Autodesk Inventor part; units mm, degrees
ref_plane "YZ Plane" through (0, 0, 0) normal (1, 0, 0) x (0, 1, 0)
ref_plane "XZ Plane" through (0, 0, 0) normal (0, 1, 0) x (-1, 0, 0)
ref_plane "XY Plane" through (0, 0, 0) normal (0, 0, 1) x (1, 0, 0)
sketch "Sketch1" plane through (0, 0, 0) normal (0, 0, 1) x (1, 0, 0)
  circle A0 centre (0, 0) radius 6.15
  line L0 (-4.2968, 4.4) -> (-16.8146, 2.7257)
  arc A1 (-16.8146, 2.7257) -> (-16.8146, -2.7257) centre (-16.45, 0) ccw
  line L1 (-16.8146, -2.7257) -> (-4.2968, -4.4)
  line L2 (4.2968, -4.4) -> (16.8146, -2.7257)
  arc A2 (16.8146, -2.7257) -> (16.8146, 2.7257) centre (16.45, 0) ccw
  line L3 (16.8146, 2.7257) -> (4.2968, 4.4)
  line L4 (-4.2968, -4.4) -> (4.2968, -4.4) construction
  line L5 (-4.2968, 4.4) -> (4.2968, 4.4) construction
  line L6 (-19.2, 0) -> (19.2, 0) construction
  circle A3 centre (0, 0) radius 11.25
  point P0 (-10.6763, 3.5467)
  point P1 (-10.6763, -3.5467)
  point P2 (10.6763, 3.5467)
  point P3 (10.6763, -3.5467)
  dimension "d0" = 12.3
  dimension "d1" = 8.8
  dimension "d2" = 38.4
  dimension "d3" = 2.75
  dimension "d10" = 22.5
extrude "Extrusion1" add sketch "Sketch1" along normal blind 2.3 contours A0 | A0 L3 A3 L2 | A0 L1 A3 L0
sketch "Sketch2" plane through (0, 0, 2.3) normal (0, 0, 1) x (1, 0, 0)
  circle A0 centre (0, 0) radius 4.4
  circle A1 centre (0, 0) radius 2.85
  dimension "d6" = 8.8
  dimension "d7" = 5.7
extrude "Extrusion2" add sketch "Sketch2" along normal blind 3.3
properties part number "attachment_real" material "Nylon 6/6"
Geometry: final body of the model. Coordinates: model frame, mm. A direction names the side the tool comes from. Coordinates: 2 decimals unless noted, no trailing zeros. Loops run counter-clockwise (first coordinate to the right, second up) from the corner with the lowest first, then second, coordinate; pieces in that order, holes last. Notation, with made-up numbers: (-38, 14) - (5, 14) arc R17 ccw to (5, 32) - close; hole circle Ø11 at (88, 88.25). An arc over 180 degrees is marked (long way). Put each result on its own line as item: value. Start each with the question number.
Q1. Cut plane A-A, the plane z = 5.05. Return loops of the section in (x, y).
Q2. Pull-direction query (Y, two-part tool) for faces 1 (the flat face through (1, -3, 5.6)), 2 (the flat face through (0, 0, 2.3)), 3 (the cylindrical face through (-0.07, 6.15, 1.13)), 4 (the cylindrical face through (-11.25, -0.05, 1.13)); classes: released by +Y, released by -Y, zero draft, split by the parting line, or undercut.
Q3. Pin query (flat end, axial travel): pin 1 Ø4 at (x, y) = (-8.5, -0.5) entering from -Z; pin 2 Ø1.5 at (x, z) = (4.5, 4) entering from +Y; pin 3 Ø2 at (x, z) = (5, 2.5) entering from -Y; pin 4 Ø2 at (x, z) = (6, 2) entering from +Y. Return the tip coordinate at first contact, or that it passes through.
Q4. Set-up query: faces 5 (the flat face through (7.44, -3.98, 1.13)), 6 (the cylindrical face through (4.197, -1.322, 3.927)). Return all of +Z, -Z, +X, -X, +Y, -Y with unobstructed straight access to the full face (end or side cutting, diameter ignored); none if empty.
Q5. Cut plane C-C, the plane y = 0. Return loops of the section in (x, z).
Q6. Cut plane D-D, the plane x = -3.5. Return loops of the section in (y, z), and give its area (3 significant figures).
Q7. Line query: line 1 (Y direction, x = 0, z = 4.7); line 2 (Z direction, x = -7.5, y = 3.25); line 3 (X direction, y = 1, z = 5.3). Output: solid intervals per line, ascending.
Q8. Cut plane B-B, the plane x = 0. Return loops of the section in (y, z).
Filled sheet:
1. outline: circle Ø8.8 at (0, 0); hole circle Ø5.7 at (0, 0)
2. face 1: zero draft
2. face 2: undercut
2. face 3: released by +Y
2. face 4: split by the parting line
3. pin 1: z = 0
3. pin 2: y = 2.3
3. pin 3: y = -4.65
3. pin 4: y = 4.31
4. face 5: +Z, -Z, +X, -Y
4. face 6: +Z
5. outline: (-11.25, 0) - (11.25, 0) - (11.25, 2.3) - (4.4, 2.3) - (4.4, 5.6) - (2.85, 5.6) - (2.85, 2.3) - (-2.85, 2.3) - (-2.85, 5.6) - (-4.4, 5.6) - (-4.4, 2.3) - (-11.25, 2.3) - close
6. outline: (-5.06, 0) - (5.06, 0) - (5.06, 2.3) - (2.67, 2.3) - (2.67, 5.6) - (-2.67, 5.6) - (-2.67, 2.3) - (-5.06, 2.3) - close
6. area: 40.9 mm²
7. line 1: -4.4 to -2.85, 2.85 to 4.4
7. line 2: 0 to 2.3
7. line 3: -4.28 to -2.67, 2.67 to 4.28
8. outline: (-6.15, 0) - (6.15, 0) - (6.15, 2.3) - (4.4, 2.3) - (4.4, 5.6) - (2.85, 5.6) - (2.85, 2.3) - (-2.85, 2.3) - (-2.85, 5.6) - (-4.4, 5.6) - (-4.4, 2.3) - (-6.15, 2.3) - close
